Could you check a few things on this model? Use its own coordinates, in mm. Round coordinates to 2 decimals unless told otherwise and drop trailing zeros. Loops run counter-clockwise (first coordinate to the right, second up) from the corner with the lowest first, then second, coordinate; pieces in that order, holes last. Notation, with made-up numbers: (2.5, 10.5) -> (20.5, 10.5) arc R24 cw to (20.5, 31.5) -> close; hole circle Ø3 at (81, 54). An arc over 180 degrees is marked (long way). Write each question's results on one line, items separated by ' | '.
Autodesk Fusion 360 part; units mm, degrees
sketch "Sketch1" plane through (0, 0, 0) normal (0, 0, 1) x (1, 0, 0)
  circle A0 centre (0, 0) radius 25.4
  circle A1 centre (0, 0) radius 22.225 construction
  line L0 (0, 0) -> (0, 25.4) construction
  circle A2 centre (0, 0) radius 15.0812 construction
  point P0 (0, 22.225)
  point P1 (0, 15.0812)
  dimension "d1" = 50.8
  dimension "d2" = 44.45
  dimension "d3" = 30.1625
extrude "Extrude1" add sketch "Sketch1" along normal blind 6.35
hole "Hole1" at (0, 0, 0) direction (0, 0, 1) diameter 4.4958 depth 6.35 tip angle 118
hole "Hole2" at (0, 15.0812, 0) direction (0, 0, 1) diameter 3.7973 depth 6.35 tip angle 118
pattern_circular "C-Pattern1" count 3 over 360 about axis through (0, 0, 0) along (0, 0, 1) of "Hole1"
pattern_circular "C-Pattern2" count 3 over 360 about axis through (0, 0, 0) along (0, 0, 1) of "Hole2"
hole "Hole3" at (0, 0, 0) direction (0, 0, 1) diameter 2.2708 depth 6.35 tip angle 180
1) I want a section at D-D, the plane x = -22. Write out the boundary of the cut face in (y, z), plus the area to 3 significant figures.
Model answer:
outline: (-12.69, 0) -> (12.69, 0) -> (12.69, 6.35) -> (-12.69, 6.35) -> close | area: 161 mm2
2) I want a section at B-B, the plane y = 0. Write out the boundary of the cut face in (x, z), plus the area to 3 significant figures.
Model answer:
outline: (-25.4, 0) -> (-2.25, 0) -> (-2.25, 6.35) -> (-25.4, 6.35) -> close; (2.25, 0) -> (25.4, 0) -> (25.4, 6.35) -> (2.25, 6.35) -> close | area: 294 mm2
3) If we mould it in two halves opening along X, with no side actions, what happens to faces 1 (the cylindrical face through (-14.943, -7.788, 3.219)), 2 (the cylindrical face through (-5.506, 24.796, 3.131)), 3 (the flat face through (5, 0, 0))? For each: released by +X, released by -X, zero draft, split by the parting line, or undercut.
Model answer:
face 1: undercut | face 2: split by the parting line | face 3: zero draft
4) I want a section at C-C, the plane z = 5.25. Write out the boundary of the cut face in (x, y).
Model answer:
outline: circle Ø50.8 at (0, 0); hole circle Ø3.8 at (-13.06, -7.54); hole circle Ø4.5 at (0, 0); hole circle Ø3.8 at (0, 15.08); hole circle Ø3.8 at (13.06, -7.54)
5) I'm going to push flat-ended pins straight in: pin 1 (3 mm diameter, centred on x = 16.5, z = 4.5, fed in from -Y); pin 2 (2 mm diameter, centred on x = -3, z = 5.5, fed in from +Y); pin 3 (2 mm diameter, centred on x = 6, z = 5.5, fed in from -Y). Where does each tip first touch, or does it pass through?
Model answer:
pin 1: stops at y = -20.5 | pin 2: stops at y = 25.32 | pin 3: stops at y = -24.9
6) I want a section at A-A, the plane x = 0. Write out the boundary of the cut face in (y, z), plus the area to 3 significant figures.
Model answer:
outline: (-25.4, 0) -> (-2.25, 0) -> (-2.25, 6.35) -> (-25.4, 6.35) -> close; (2.25, 0) -> (13.18, 0) -> (13.18, 6.35) -> (2.25, 6.35) -> close; (16.98, 0) -> (25.4, 0) -> (25.4, 6.35) -> (16.98, 6.35) -> close | area: 270 mm2
7) I need wall thicknesses on line 1 (Y direction, x = 0, z = 3.25); line 2 (Y direction, x = -1.5, z = 4); line 3 (X direction, y = -7.5, z = 2). Which ranges of each line are inside material? Lowest first, please.
Model answer:
line 1: y = -25.4 to -2.25, 2.25 to 13.18, 16.98 to 25.4 | line 2: y = -25.36 to -1.67, 1.67 to 13.92, 16.25 to 25.36 | line 3: x = -24.27 to -14.96, -11.16 to 11.16, 14.96 to 24.27
